Geometry check sheet. Reference: the model listing, model coordinates, mm. A direction names the side the tool comes from. Round coordinates to 2 decimals unless told otherwise and drop trailing zeros. Write each loop counter-clockwise with the first axis right and the second up, starting at its lowest first coordinate (ties: lowest second). Pieces come first, ordered by that corner, then holes. Notation, with made-up numbers: M 63.25,59 L 98.25,59 A7 ccw 98.25,68 Z; hole C -24,37 d10. An arc over 180 degrees is marked long. Use a Markdown table: item, result.
```python
from build123d import *

# Parameters (mm, degrees)
SKETCH1_R                       = 57.5945
EXTRUDE1_DEPTH                  = 10.16
SKETCH2_R                       = 54.5465
EXTRUDE2_DEPTH                  = 4.826
F_1_4_0_25_DIAMETER_HOLE1_D     = 6.35
F_1_4_0_25_DIAMETER_HOLE1_DEPTH = 6.35
F_1_4_0_25_DIAMETER_HOLE1_TIP   = 1.907732465
F_1_4_CLEARANCE_HOLE1_D         = 7.14248
CIRPATTERN1_COUNT               = 4


with BuildPart() as part:
    # Sketch1 → Extrude1 (new body)
    with BuildSketch(Plane.XY):
        Circle(SKETCH1_R)
    extrude(amount=EXTRUDE1_DEPTH)

    # Sketch2 → Extrude2 (cut)
    with BuildSketch(Plane.XY.offset(10.16)):
        Circle(SKETCH2_R)
    extrude(amount=-EXTRUDE2_DEPTH, mode=Mode.SUBTRACT)

    # 1/4 (0.25) Diameter Hole1
    with Locations(Plane.XY.offset(5.334)):
        with Locations((0, 0)):
            Hole(F_1_4_0_25_DIAMETER_HOLE1_D / 2, depth=F_1_4_0_25_DIAMETER_HOLE1_DEPTH)
            with Locations((0, 0, -(F_1_4_0_25_DIAMETER_HOLE1_DEPTH + F_1_4_0_25_DIAMETER_HOLE1_TIP / 2))):  # 118° drill point
                Cone(0, F_1_4_0_25_DIAMETER_HOLE1_D / 2, F_1_4_0_25_DIAMETER_HOLE1_TIP, mode=Mode.SUBTRACT)

    # 1/4 Clearance Hole1 (through all)
    with Locations(Plane(origin=(25.4, 0, 5.334), x_dir=(1, 0, 0), z_dir=(0, 0, 1))):
        with Locations((0, 0)):
            f_1_4_clearance_hole1 = Hole(F_1_4_CLEARANCE_HOLE1_D / 2)

    # CirPattern1: 1/4 Clearance Hole1 ×4 about axis
    cirpattern1_axis = Axis((0, 0, 0), (0, 0, 1))
    for i in range(1, CIRPATTERN1_COUNT):
        add(f_1_4_clearance_hole1.rotate(cirpattern1_axis, i * 360 / CIRPATTERN1_COUNT), mode=Mode.SUBTRACT)


solid = part.part
```
Item 1: Cross-section at D-D, the plane y = -46.5. Record the cut outline in (x, z), and give its area (3 significant figures).
Outcome:
| item | result |
|---|---|
| outline | M -33.98,0 L 33.98,0 L 33.98,10.16 L 28.51,10.16 L 28.51,5.33 L -28.51,5.33 L -28.51,10.16 L -33.98,10.16 Z |
| area | 415 mm2 |
Item 2: Go/stop test with flat-tipped pins: pin 1 (1.5 mm diameter, centred on x = 12.5, z = 2, fed in from +Y); pin 2 (2 mm diameter, centred on x = 26.5, z = 8.5, fed in from +Y); pin 3 (2 mm diameter, centred on y = 44.5, z = 7, fed in from +X). Record where each tip stops, or that it passes through.
Outcome:
| item | result |
|---|---|
| pin 1 | stops at y = 56.38 |
| pin 2 | stops at y = 51.64 |
| pin 3 | stops at x = 37.75 |
Item 3: Mould release check, pull along X, two halves, no side actions. Record for faces 3 (the face through (-28.968, -0.157, 2.63)), 4 (the face through (-1, -12, 0)), 5 (the face through (-7.498, 57.104, 5.009)): +X half, -X half, draft (parallel to the pull), parting line (faces both ways), or undercut.
Outcome:
| item | result |
|---|---|
| face 3 | undercut |
| face 4 | draft |
| face 5 | parting line |
Item 4: Cross-section at A-A, the plane x = 0. Record the cut outline in (y, z) (1 decimal).
Outcome:
| item | result |
|---|---|
| outline | M -57.6,0 L -29,0 L -29,5.3 L -54.5,5.3 L -54.5,10.2 L -57.6,10.2 Z; M -21.8,0 L -3.2,0 L -3.2,5.3 L -21.8,5.3 Z; M 3.2,0 L 21.8,0 L 21.8,5.3 L 3.2,5.3 Z; M 29,0 L 57.6,0 L 57.6,10.2 L 54.5,10.2 L 54.5,5.3 L 29,5.3 Z |
Item 5: Cross-section at C-C, the plane x = 24. Record the cut outline in (y, z).
Outcome:
| item | result |
|---|---|
| outline | M -52.36,0 L -3.29,0 L -3.29,5.33 L -48.98,5.33 L -48.98,10.16 L -52.36,10.16 Z; M 3.29,0 L 52.36,0 L 52.36,10.16 L 48.98,10.16 L 48.98,5.33 L 3.29,5.33 Z |
Item 6: Cross-section at B-B, the plane y = -25.4. Record the cut outline in (x, z).
Outcome:
| item | result |
|---|---|
| outline | M -51.69,0 L -3.57,0 L -3.57,5.33 L -48.27,5.33 L -48.27,10.16 L -51.69,10.16 Z; M 3.57,0 L 51.69,0 L 51.69,10.16 L 48.27,10.16 L 48.27,5.33 L 3.57,5.33 Z |
Item 7: Material ranges on line 1 along Y through (x, z) = (-6, 8); line 2 along Z through (x, y) = (1, 36); line 3 along Y through (x, z) = (19, 6), recorded low to high. Write a range as from..to.
Outcome:
| item | result |
|---|---|
| line 1 | y = -57.28..-54.22, 54.22..57.28 |
| line 2 | z = 0..5.33 |
| line 3 | y = -54.37..-51.13, 51.13..54.37 |
Item 8: Access from +Z, -Z, +X, -X, +Y, -Y to the whole of each face (thin tool, end or side, straight path). Record for faces 1 (the face through (52.03, 16.38, 7.78)), 2 (the face through (0.69, -3.1, 2.63)).
Outcome:
| item | result |
|---|---|
| face 1 | +Z |
| face 2 | +Z, -Z |
